Verification items for the finished model (mm, model axes). Coordinates: 2 decimals unless noted, no trailing zeros. Order: outer loops, then holes, each group sorted by start corner. A loop starts at its lowest first (then second) coordinate and runs counter-clockwise, first axis right, second up. Notation, with made-up numbers: M 7.5,43 L 53.5,43 A12 cw 53.5,48 Z; hole C -12.75,25 d4. An arc over 180 degrees is marked long. Write item = value, one per line.
```python
from build123d import *

# Parameters (mm, degrees)
F1_DEPTH = 1.016
F2_DEPTH = 1.0170001
F3_R     = 1.27


with BuildPart() as f1:
    # F0 (on Top) → F1 (new body, symmetric)
    with BuildSketch(Plane.XY):
        with BuildLine():
            ThreePointArc((45.6495498851, -23.422840547), (49.8733293931, -12.0483143738), (51.308, 0))
            ThreePointArc((51.308, 0), (37.1674130388, 35.370811017), (2.54, 51.2450901453))
            Line((2.54, 51.2450901453), (-2.54, 51.2450901453))
            ThreePointArc((-2.54, 51.2450901453), (-44.4340314174, 25.654), (-45.6495498851, -23.422840547))
            Line((-45.6495498851, -23.422840547), (-43.1095498851, -27.8222495983))
            ThreePointArc((-43.1095498851, -27.8222495983), (0, -51.308), (43.1095498851, -27.8222495983))
            Line((43.1095498851, -27.8222495983), (45.6495498851, -23.422840547))
        make_face()
        with BuildLine():
            add(Edge.make_bspline(
                [(0, -8.89), (10.9985226281, -8.89), (5.499261314, 4.445), (0, 17.78), (-5.499261314, 4.445), (-10.9985226281, -8.89), (0, -8.89)],
                knots=[0, 0, 0, 2.0943951024, 2.0943951024, 4.1887902048, 4.1887902048, 6.2831853072, 6.2831853072, 6.2831853072], degree=2, weights=[1, 0.5, 1, 0.5, 1, 0.5, 1]))
        make_face(mode=Mode.SUBTRACT)
        with BuildLine():
            Line((-2.54, 51.2450901453), (2.54, 51.2450901453))
            ThreePointArc((2.54, 51.2450901453), (0, 51.308), (-2.54, 51.2450901453))
        make_face()
        with BuildLine():
            ThreePointArc((-2.54, 51.2450901453), (0, 51.308), (2.54, 51.2450901453))
            Line((2.54, 51.2450901453), (2.54, 56.3250901453))
            Line((2.54, 56.3250901453), (-2.54, 56.3250901453))
            Line((-2.54, 56.3250901453), (-2.54, 51.2450901453))
        make_face()
        with BuildLine():
            Line((50.0489589363, -25.962840547), (45.6495498851, -23.422840547))
            ThreePointArc((45.6495498851, -23.422840547), (44.4340314174, -25.654), (43.1095498851, -27.8222495983))
            Line((43.1095498851, -27.8222495983), (47.5089589363, -30.3622495983))
            Line((47.5089589363, -30.3622495983), (50.0489589363, -25.962840547))
        make_face()
        with BuildLine():
            ThreePointArc((43.1095498851, -27.8222495983), (44.4340314174, -25.654), (45.6495498851, -23.422840547))
            Line((45.6495498851, -23.422840547), (43.1095498851, -27.8222495983))
        make_face()
        with BuildLine():
            Line((-43.1095498851, -27.8222495983), (-45.6495498851, -23.422840547))
            ThreePointArc((-45.6495498851, -23.422840547), (-44.4340314174, -25.654), (-43.1095498851, -27.8222495983))
        make_face()
        with BuildLine():
            ThreePointArc((-43.1095498851, -27.8222495983), (-44.4340314174, -25.654), (-45.6495498851, -23.422840547))
            Line((-45.6495498851, -23.422840547), (-50.0489589363, -25.962840547))
            Line((-50.0489589363, -25.962840547), (-47.5089589363, -30.3622495983))
            Line((-47.5089589363, -30.3622495983), (-43.1095498851, -27.8222495983))
        make_face()
    extrude(amount=F1_DEPTH, both=True)

    # F0 (on Top) → F2 (cut, through all)
    with BuildSketch(Plane.XY):
        with BuildLine():
            ThreePointArc((45.6495498851, -23.422840547), (49.8733293931, -12.0483143738), (51.308, 0))
            ThreePointArc((51.308, 0), (37.1674130388, 35.370811017), (2.54, 51.2450901453))
            Line((2.54, 51.2450901453), (-2.54, 51.2450901453))
            ThreePointArc((-2.54, 51.2450901453), (-44.4340314174, 25.654), (-45.6495498851, -23.422840547))
            Line((-45.6495498851, -23.422840547), (-43.1095498851, -27.8222495983))
            ThreePointArc((-43.1095498851, -27.8222495983), (0, -51.308), (43.1095498851, -27.8222495983))
            Line((43.1095498851, -27.8222495983), (45.6495498851, -23.422840547))
        make_face()
        with BuildLine():
            add(Edge.make_bspline(
                [(0, -8.89), (10.9985226281, -8.89), (5.499261314, 4.445), (0, 17.78), (-5.499261314, 4.445), (-10.9985226281, -8.89), (0, -8.89)],
                knots=[0, 0, 0, 2.0943951024, 2.0943951024, 4.1887902048, 4.1887902048, 6.2831853072, 6.2831853072, 6.2831853072], degree=2, weights=[1, 0.5, 1, 0.5, 1, 0.5, 1]))
        make_face(mode=Mode.SUBTRACT)
        with BuildLine():
            Line((-2.54, 51.2450901453), (2.54, 51.2450901453))
            ThreePointArc((2.54, 51.2450901453), (0, 51.308), (-2.54, 51.2450901453))
        make_face()
        with BuildLine():
            ThreePointArc((-2.54, 51.2450901453), (0, 51.308), (2.54, 51.2450901453))
            Line((2.54, 51.2450901453), (2.54, 56.3250901453))
            Line((2.54, 56.3250901453), (-2.54, 56.3250901453))
            Line((-2.54, 56.3250901453), (-2.54, 51.2450901453))
        make_face()
        with BuildLine():
            Line((50.0489589363, -25.962840547), (45.6495498851, -23.422840547))
            ThreePointArc((45.6495498851, -23.422840547), (44.4340314174, -25.654), (43.1095498851, -27.8222495983))
            Line((43.1095498851, -27.8222495983), (47.5089589363, -30.3622495983))
            Line((47.5089589363, -30.3622495983), (50.0489589363, -25.962840547))
        make_face()
        with BuildLine():
            ThreePointArc((43.1095498851, -27.8222495983), (44.4340314174, -25.654), (45.6495498851, -23.422840547))
            Line((45.6495498851, -23.422840547), (43.1095498851, -27.8222495983))
        make_face()
        with BuildLine():
            Line((-43.1095498851, -27.8222495983), (-45.6495498851, -23.422840547))
            ThreePointArc((-45.6495498851, -23.422840547), (-44.4340314174, -25.654), (-43.1095498851, -27.8222495983))
        make_face()
        with BuildLine():
            ThreePointArc((-43.1095498851, -27.8222495983), (-44.4340314174, -25.654), (-45.6495498851, -23.422840547))
            Line((-45.6495498851, -23.422840547), (-50.0489589363, -25.962840547))
            Line((-50.0489589363, -25.962840547), (-47.5089589363, -30.3622495983))
            Line((-47.5089589363, -30.3622495983), (-43.1095498851, -27.8222495983))
        make_face()
    extrude(amount=-F2_DEPTH, mode=Mode.SUBTRACT)

    # F3
    f3_edges = [f1.edges().sort_by_distance(p)[0] for p in [
        (-50.048959, -25.962841, 0.508),
        (-47.508959, -30.36225, 0.508),
        (2.54, 56.32509, 0.508),
        (-2.54, 56.32509, 0.508),
        (50.048959, -25.962841, 0.508),
        (47.508959, -30.36225, 0.508),
    ]]
    fillet(f3_edges, radius=F3_R)


solid = f1.part
```
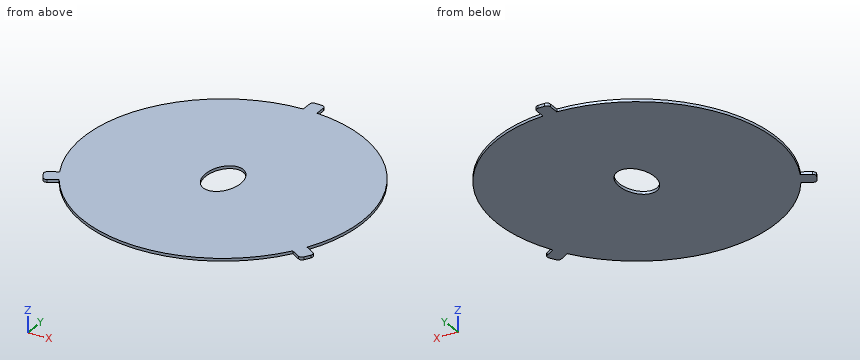
Item 1: Sectioned sample at B-B, the plane x = -31.5. Enter the section's corners in (y, z).
Report:
outline = M -40.5,0 L 40.5,0 L 40.5,1.02 L -40.5,1.02 Z
Item 2: Scan lines: L1, parallel to X at y = 5.5, z = 0.3; L2, parallel to X at y = -10.5, z = 0.4; L3, parallel to X at y = -3, z = 0.45. Record each from-to range of solid material in increasing order. Write a range as from..to.
Report:
L1 = -51.01..-4.99, 4.99..51.01
L2 = -50.22..50.22
L3 = -51.22..-5.98, 5.98..51.22
Item 3: Sectioned sample at A-A, the plane y = -35. Enter the section's corners in (x, z), then the cut area to 3 significant figures.
Report:
outline = M -37.52,0 L 37.52,0 L 37.52,1.02 L -37.52,1.02 Z
area = 76.2 mm^2
